```python
from build123d import *

# Parameters (mm, degrees)
SKETCH1_R           = 5
BOSS_EXTRUDE1_DEPTH = 10
SKETCH2_R           = 10
BOSS_EXTRUDE2_DEPTH = 1
BOSS_EXTRUDE3_DEPTH = 5


with BuildPart() as part:
    # Sketch1 → Boss-Extrude1 (new body)
    with BuildSketch(Plane.XY):
        with BuildLine():
            Line((12, 2), (12, -2))
            Line((12, -2), (9.797958971, -2))
            ThreePointArc((9.797958971, -2), (-10, 0), (9.797958971, 2))
            Line((9.797958971, 2), (12, 2))
        make_face()
        Circle(SKETCH1_R, mode=Mode.SUBTRACT)
    extrude(amount=BOSS_EXTRUDE1_DEPTH)

    # Sketch2 → Boss-Extrude2 (add)
    with BuildSketch(Plane.XY.offset(10)):
        with Locations(Location((0, 0, 0), (0, 0, 348.463040967))):
            Circle(SKETCH2_R)
    extrude(amount=BOSS_EXTRUDE2_DEPTH)

    # Sketch3 → Boss-Extrude3 (add)
    with BuildSketch(Plane.XY.offset(11)):
        Polygon((4.618802154, 0), (2.309401077, 4), (-2.309401077, 4), (-4.618802154, 0), (-2.309401077, -4), (2.309401077, -4), align=None)
    extrude(amount=BOSS_EXTRUDE3_DEPTH)


solid = part.part
```
Geometry check sheet. Reference: the model listing, model coordinates, mm. A direction names the side the tool comes from. Give positions to 0.01 mm unless a question says otherwise; leave off trailing zeros. Write each loop counter-clockwise with the first axis right and the second up, starting at its lowest first coordinate (ties: lowest second). Pieces come first, ordered by that corner, then holes.
1) Section check D-D, the plane z = 14. Record the boundary of the cut face in (x, y).
2) Section check B-B, the plane z = 6.5. Record the boundary of the cut face in (x, y).
3) Material ranges on L1, parallel to Y at x = 0, z = 7; L2, parallel to X at y = -4, z = 5.75; L3, parallel to Y at x = -2.25, z = 14.75, recorded low to high.
4) Section check C-C, the plane x = 0. Record the boundary of the cut face in (y, z), and give its area (3 significant figures).
5) Gauge pin test, flat ends, axial feed: pin 1 (5 mm diameter, centred on x = 0.5, z = 13, fed in from -Y); pin 2 (2 mm diameter, centred on y = 4.5, z = 2.5, fed in from -X); pin 3 (5 mm diameter, centred on x = 1.5, z = 14, fed in from +Y); pin 4 (0.7 mm diameter, centred on x = 11.5, y = 0, fed in from +Z). Record the tip position at first contact, or that the pin passes through.
6) Section check A-A, the plane y = -6. Record the boundary of the cut face in (x, z), and give its area (3 significant figures).
7) Release check for a two-part mould opening along Y. For faces 6 (the flat face through (-3.448, 2.028, 13.465)), 7 (the flat face through (0, 0, 10)), 8 (the cylindrical face through (-1.08, -4.88, 4.93)), 9 (the flat face through (4, -4, 0)) record: pulls with the +Y half, pulls with the -Y half, needs draft (parallel to the pull), parting line crosses it, or undercut.
8) Access from +Z, -Z, +X, -X, +Y, -Y to the whole of each face (thin tool, end or side, straight path). Record for faces 1 (the flat face through (3.48, 1.97, 13.46)), 2 (the flat face through (3.448, -2.028, 13.465)), 3 (the flat face through (-3.48, -1.97, 13.46)), 4 (the flat face through (11, 2, 5)), 5 (the flat face through (0, -4, 13)).
Computed:
1. outline: (-4.62, 0) - (-2.31, -4) - (2.31, -4) - (4.62, 0) - (2.31, 4) - (-2.31, 4) - close
2. outline: (9.8, -2) - (12, -2) - (12, 2) - (9.8, 2) arc R10 ccw (long way) to start; hole circle Ø10 at (0, 0)
3. L1: y = -10 to -5, 5 to 10
3. L2: x = -9.17 to -3, 3 to 9.17
3. L3: y = -4 to 4
4. outline: (-10, 0) - (-5, 0) - (-5, 10) - (5, 10) - (5, 0) - (10, 0) - (10, 11) - (4, 11) - (4, 16) - (-4, 16) - (-4, 11) - (-10, 11) - close
4. area: 160 mm2
5. pin 1: stops at y = -10
5. pin 2: stops at x = -9.37
5. pin 3: stops at y = 4
5. pin 4: stops at z = 10
6. outline: (-8, 0) - (8, 0) - (8, 11) - (-8, 11) - close
6. area: 176 mm2
7. face 6: pulls with the +Y half
7. face 7: undercut
7. face 8: undercut
7. face 9: needs draft
8. face 1: +Z, +X, +Y
8. face 2: +Z, +X, -Y
8. face 3: +Z, -X, -Y
8. face 4: +Z, -Z, +X, +Y
8. face 5: +Z, +X, -X, -Y
